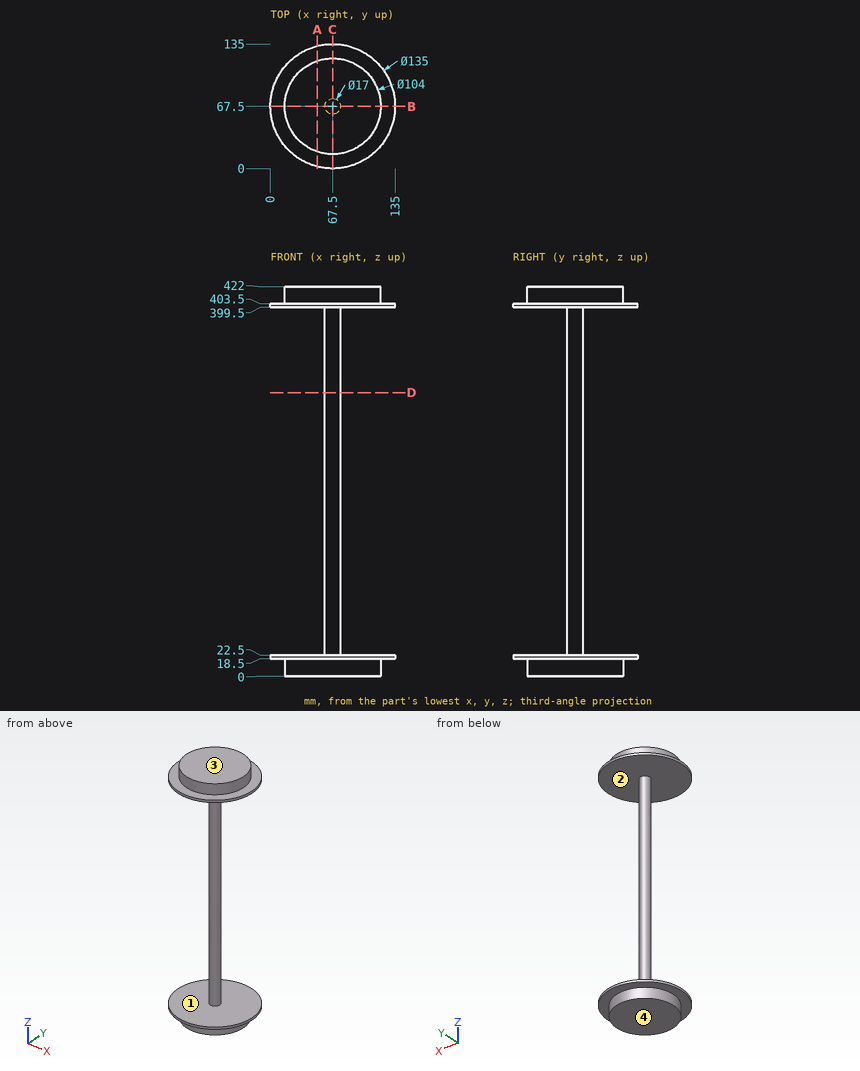
Geometry check sheet. Reference: drawing and pictorial views, mm from the part's lowest x, y, z. Coordinates: 2 decimals unless noted, no trailing zeros. Write each loop counter-clockwise with the first axis right and the second up, starting at its lowest first coordinate (ties: lowest second). Pieces come first, ordered by that corner, then holes. Notation, with made-up numbers: (70, -35.5) - (119, -35.5) arc R14 ccw to (119, -16.5) - close; hole circle Ø8 at (12, -19.5). An arc over 180 degrees is marked (long way). Write item = value, one per line.
Q1. Cross-section at B-B (y = 67.5). Enter the section's corners in (x, z).
Answer:
outline = (0, 18.5) - (15.5, 18.5) - (15.5, 0) - (119.5, 0) - (119.5, 18.5) - (135, 18.5) - (135, 22.5) - (76, 22.5) - (76, 399.5) - (135, 399.5) - (135, 403.5) - (119.5, 403.5) - (119.5, 422) - (15.5, 422) - (15.5, 403.5) - (0, 403.5) - (0, 399.5) - (59, 399.5) - (59, 22.5) - (0, 22.5) - close
Q2. Cross-section at A-A (x = 51). Enter the section's corners in (y, z), plus the area to 3 significant figures.
Answer:
outline = (2.05, 18.5) - (18.19, 18.5) - (18.19, 0) - (116.81, 0) - (116.81, 18.5) - (132.95, 18.5) - (132.95, 22.5) - (2.05, 22.5) - close; (2.05, 399.5) - (132.95, 399.5) - (132.95, 403.5) - (116.81, 403.5) - (116.81, 422) - (18.19, 422) - (18.19, 403.5) - (2.05, 403.5) - close
area = 4,700 mm²
Q3. Go/stop test with flat-tipped pins: pin 1 Ø2 at (x, y) = (30.5, 25) entering from +Z; pin 2 Ø6 at (x, y) = (102.5, 20) entering from -Z; pin 3 Ø12 at (x, y) = (84, 102) entering from -Z. Record where each tip stops, or that it passes through.
Answer:
pin_1 = 403.5
pin_2 = 18.5
pin_3 = 0
Q4. Cross-section at D-D (z = 307). Enter the section's corners in (x, y), plus the area to 3 significant figures.
Answer:
outline = circle Ø17 at (67.5, 67.5)
area = 227 mm²
Q5. Material ranges on L1, parallel to Z at x = 118, y = 50; L2, parallel to Z at x = 77, y = 106; L3, parallel to X at y = 75, z = 107, recorded low to high. Write a range as from..to.
Answer:
L1 = 18.5..22.5, 399.5..403.5
L2 = 0..22.5, 399.5..422
L3 = 63.5..71.5
Q6. Mould release check, pull along Z, two halves, no side actions. Record for the marked faces 1, 2, 3 and 4: released by +Z, released by -Z, zero draft, split by the parting line, or undercut.
Answer:
face_1 = undercut
face_2 = undercut
face_3 = released by +Z
face_4 = released by -Z
